Input: part model. Units: mm. Frame: model coordinates. A direction names the side the tool comes from. Round coordinates to 2 decimals unless told otherwise and drop trailing zeros. Loops run counter-clockwise (first coordinate to the right, second up) from the corner with the lowest first, then second, coordinate; pieces in that order, holes last. Notation, with made-up numbers: M 19,-6 L 33,-6 A16 ccw 33,23 Z; hole C -37.5,-16.5 d11. An arc over 180 degrees is marked long. Put each result on its own line as item: value. Start each with the question number.
1) Section A-A on x = 70. Output: boundary loops of the cut face in (y, z), plus the area to 3 significant figures.
2) Section C-C on z = 1.3. State how many separate pieces and enclosed holes the cut face has, plus the area to 3 significant figures.
3) Draft query along X for faces 3 (the face through (31.666, -38.722, 1.521)), 4 (the face through (-80, -13, 1)), 5 (the face through (80, -1, 1)), 6 (the face through (17, 1, 3)). Return one class per face: +X half, -X half, draft (parallel to the pull), parting line (faces both ways), or undercut.
4) Pin query (flat end, axial travel): pin 1 (2 mm diameter, centred on x = 7.5, y = 6.5, fed in from +Z); pin 2 (1.5 mm diameter, centred on y = 40.5, z = 1.5, fed in from -X); pin 3 (1.5 mm diameter, centred on x = -65, z = 1, fed in from +Y). Return the tip coordinate at first contact, or that it passes through.
5) Section B-B on y = -40. Output: boundary loops of the cut face in (x, z), plus the area to 3 significant figures.
6) Line query: probe 1 along Y at (x, z) = (0, 0.7); probe 2 along Y at (x, z) = (-70, 1.65); probe 3 along Y at (x, z) = (30, 0.7). Output: solid intervals per line, ascending.
7) Reachability of faces 1 (the face through (-69, 27, 1)), 2 (the face through (12, 50, 1)) from +Z, -Z, +X, -X, +Y, -Y: full face, straight path, thin tool, end or side. Return the list, or none.
8) Section D-D on x = -70. Output: boundary loops of the cut face in (y, z), plus the area to 3 significant figures.
from build123d import *

# Parameters (mm, degrees)
SKETCH_1_W               = 160
SKETCH_1_H               = 100
EXTRUDE_1_DEPTH          = 3
SKETCH_2_R               = 2.1
CUT_EXTRUDE_1_DEPTH      = 95.387499172
CUT_EXTRUDE_2_DEPTH      = 95.387499172
CUT_EXTRUDE_2_DEPTH_BACK = 95.387499172
SKETCH_3_R               = 1.25
CUT_EXTRUDE_3_DEPTH      = 95.387499172
CUT_EXTRUDE_3_DEPTH_BACK = 95.387499172
SKETCH_4_R               = 12.5
CUT_EXTRUDE_4_DEPTH      = 95.387499172
CUT_EXTRUDE_4_DEPTH_BACK = 95.387499172
SKETCH_5_W               = 23
SKETCH_5_H               = 23
FILLET_1_R               = 2


with BuildPart() as part:
    # 草图1 → 凸台-拉伸1 (new body)
    with BuildSketch(Plane.XY):
        Rectangle(SKETCH_1_W, SKETCH_1_H)
    extrude(amount=EXTRUDE_1_DEPTH)

    # 草图2 → 切除-拉伸1 (cut, through all)
    with BuildSketch(Plane.XY.offset(3)):
        with Locations((-70, 40)):
            Circle(SKETCH_2_R)
        with Locations((-30, 40)):
            Circle(SKETCH_2_R)
        with Locations((0, 40)):
            Circle(SKETCH_2_R)
        with Locations((30, 40)):
            Circle(SKETCH_2_R)
        with Locations((70, 40)):
            Circle(SKETCH_2_R)
        with Locations((-70, 0)):
            Circle(SKETCH_2_R)
        with Locations((-70, -40)):
            Circle(SKETCH_2_R)
        with Locations((-70, -80)):
            Circle(SKETCH_2_R)
        with Locations((-70, -120)):
            Circle(SKETCH_2_R)
        with Locations((-70, -160)):
            Circle(SKETCH_2_R)
        with Locations((-70, -200)):
            Circle(SKETCH_2_R)
        with Locations((-70, -240)):
            Circle(SKETCH_2_R)
        with Locations((-70, -280)):
            Circle(SKETCH_2_R)
        with Locations((70, -280)):
            Circle(SKETCH_2_R)
        with Locations((70, -240)):
            Circle(SKETCH_2_R)
        with Locations((70, -200)):
            Circle(SKETCH_2_R)
        with Locations((70, -160)):
            Circle(SKETCH_2_R)
        with Locations((70, -120)):
            Circle(SKETCH_2_R)
        with Locations((70, -80)):
            Circle(SKETCH_2_R)
        with Locations(Location((70, -40, 0), (0, 0, 180))):
            Circle(SKETCH_2_R)
        with Locations(Location((70, 0, 0), (0, 0, 180))):
            Circle(SKETCH_2_R)
        with Locations(Location((30, -40, 0), (0, 0, 180))):
            Circle(SKETCH_2_R)
        with Locations(Location((0, -40, 0), (0, 0, 180))):
            Circle(SKETCH_2_R)
        with Locations(Location((-30, -40, 0), (0, 0, 180))):
            Circle(SKETCH_2_R)
    extrude(amount=-CUT_EXTRUDE_1_DEPTH, mode=Mode.SUBTRACT)

    # 草图3 → 切除-拉伸2 (cut, two sides: drawn at the far end of the back side and taken through both)
    with BuildSketch(Plane(origin=(0, 0, 0), x_dir=(-1, 0, 0), z_dir=(0, 0, -1)).offset(-CUT_EXTRUDE_2_DEPTH_BACK)):
        with Locations((19, 0)):
            Circle(SKETCH_3_R)
        with Locations((0, -19)):
            Circle(SKETCH_3_R)
        with Locations((-19, 0)):
            Circle(SKETCH_3_R)
        with Locations((0, 19)):
            Circle(SKETCH_3_R)
    extrude(amount=CUT_EXTRUDE_2_DEPTH + CUT_EXTRUDE_2_DEPTH_BACK, mode=Mode.SUBTRACT)

    # 草图4 → 切除-拉伸3 (cut, two sides: drawn at the far end of the back side and taken through both)
    with BuildSketch(Plane(origin=(0, 0, 0), x_dir=(-1, 0, 0), z_dir=(0, 0, -1)).offset(-CUT_EXTRUDE_3_DEPTH_BACK)):
        Circle(SKETCH_4_R)
    extrude(amount=CUT_EXTRUDE_3_DEPTH + CUT_EXTRUDE_3_DEPTH_BACK, mode=Mode.SUBTRACT)

    # 草图5 → 切除-拉伸4 (cut, two sides: drawn at the far end of the back side and taken through both)
    with BuildSketch(Plane.XY.offset(3).offset(-CUT_EXTRUDE_4_DEPTH_BACK)):
        with Locations((-68.5, 38.5)):
            Rectangle(SKETCH_5_W, SKETCH_5_H)
    extrude(amount=CUT_EXTRUDE_4_DEPTH + CUT_EXTRUDE_4_DEPTH_BACK, mode=Mode.SUBTRACT)

    # 圆角1
    fillet_1_edges = [part.edges().sort_by_distance(p)[0] for p in [
        (-80, 27, 1.5),
        (-57, 50, 1.5),
        (-57, 27, 1.5),
    ]]
    fillet(fillet_1_edges, radius=FILLET_1_R)


solid = part.part
Geometry results:
1. outline: M -50,0 L -42.1,0 L -42.1,3 L -50,3 Z; M -37.9,0 L -2.1,0 L -2.1,3 L -37.9,3 Z; M 2.1,0 L 37.9,0 L 37.9,3 L 2.1,3 Z; M 42.1,0 L 50,0 L 50,3 L 42.1,3 Z
1. area: 262 mm²
2. separate pieces: 1
2. enclosed holes: 16
2. area: 14,800 mm²
3. face 3: undercut
3. face 4: -X half
3. face 5: +X half
3. face 6: draft
4. pin 1: passes through
4. pin 2: stops at x = -57
4. pin 3: stops at y = 27
5. outline: M -80,0 L -72.1,0 L -72.1,3 L -80,3 Z; M -67.9,0 L -32.1,0 L -32.1,3 L -67.9,3 Z; M -27.9,0 L -2.1,0 L -2.1,3 L -27.9,3 Z; M 2.1,0 L 27.9,0 L 27.9,3 L 2.1,3 Z; M 32.1,0 L 67.9,0 L 67.9,3 L 32.1,3 Z; M 72.1,0 L 80,0 L 80,3 L 72.1,3 Z
5. area: 417 mm²
6. probe 1: y = -50 to -42.1, -37.9 to -20.25, -17.75 to -12.5, 12.5 to 17.75, 20.25 to 37.9, 42.1 to 50
6. probe 2: y = -50 to -42.1, -37.9 to -2.1, 2.1 to 27
6. probe 3: y = -50 to -42.1, -37.9 to 37.9, 42.1 to 50
7. face 1: +Z, -Z, -X, +Y
7. face 2: +Z, -Z, +X, -X, +Y
8. outline: M -50,0 L -42.1,0 L -42.1,3 L -50,3 Z; M -37.9,0 L -2.1,0 L -2.1,3 L -37.9,3 Z; M 2.1,0 L 27,0 L 27,3 L 2.1,3 Z
8. area: 206 mm²
